```python
from build123d import *

# Parameters (mm, degrees)
SKETCH1_W               = 76.2
SKETCH1_H               = 25.4
SKETCH1_W_2             = 69.85
SKETCH1_H_2             = 19.05
EXTRUDE_THIN1_DEPTH     = 73.025
SKETCH2_W               = 63.5
SKETCH2_H               = 12.7
CUT_EXTRUDE1_DEPTH      = 26.4
SKETCH3_R               = 2.4892
CUT_EXTRUDE2_DEPTH      = 1
CUT_EXTRUDE2_DEPTH_BACK = 77.2
SKETCH4_R               = 6.35
CUT_EXTRUDE3_DEPTH      = 26.4


with BuildPart() as part:
    # Sketch1 → Extrude-Thin1 (new body, symmetric)
    with BuildSketch(Plane.XY):
        Rectangle(SKETCH1_W, SKETCH1_H)
        Rectangle(SKETCH1_W_2, SKETCH1_H_2, mode=Mode.SUBTRACT)
    extrude(amount=EXTRUDE_THIN1_DEPTH, both=True)

    # Sketch2 → Cut-Extrude1 (cut, through all)
    with BuildSketch(Plane.XZ.offset(12.7)):
        with Locations((0, -66.675)):
            Rectangle(SKETCH2_W, SKETCH2_H)
        with Locations((0, 66.675)):
            Rectangle(SKETCH2_W, SKETCH2_H)
    extrude(amount=-CUT_EXTRUDE1_DEPTH, mode=Mode.SUBTRACT)

    # Sketch3 → Cut-Extrude2 (cut, two sides)
    with BuildSketch(Plane(origin=(38.1, 0, 0), x_dir=(0, 0, -1), z_dir=(1, 0, 0))) as cut_extrude2_sk:
        with Locations((60.325, 7.62)):
            Circle(SKETCH3_R)
        with Locations((34.925, 7.62)):
            Circle(SKETCH3_R)
        with Locations((-34.925, 7.62)):
            Circle(SKETCH3_R)
        with Locations((-60.325, 7.62)):
            Circle(SKETCH3_R)
    extrude(amount=CUT_EXTRUDE2_DEPTH, mode=Mode.SUBTRACT)
    extrude(cut_extrude2_sk.sketch, amount=-CUT_EXTRUDE2_DEPTH_BACK, mode=Mode.SUBTRACT)

    # Sketch4 → Cut-Extrude3 (cut, through all)
    with BuildSketch(Plane.XZ.offset(12.7)):
        with Locations((0, 9.525)):
            Circle(SKETCH4_R)
    extrude(amount=-CUT_EXTRUDE3_DEPTH, mode=Mode.SUBTRACT)


solid = part.part
```
The listing builds one solid part. Answer for the finished solid, in the listing's coordinates (mm). A direction names the side the tool comes from. Round coordinates to 2 decimals unless told otherwise and drop trailing zeros. Write each loop counter-clockwise with the first axis right and the second up, starting at its lowest first coordinate (ties: lowest second). Pieces come first, ordered by that corner, then holes. Notation, with made-up numbers: (3.25, -19) -> (29.25, -19) arc R23 ccw to (29.25, 11) -> close; hole circle Ø10 at (52, -38). An arc over 180 degrees is marked (long way). Use CSV: the item, a comma, the result in double quotes. Start each with the question number.
(1) Section A-A on x = 0 is taken. Give the vertices of the cut face in (y, z) (3 decimals).
(2) Section B-B on z = -49 is taken. Give the vertices of the cut face in (x, y) (3 decimals).
(3) Each of these flat-tipped pins is pushed along its axis until it touches: pin 1 (1.6 mm diameter, centred on x = 1.5, y = -11.5, fed in from +Z) (3 decimals); pin 2 (0.8 mm diameter, centred on x = -9, y = 11.5, fed in from -Z) (3 decimals). Where does it stop, or does it pass through?
(4) Which of the six approach directions +Z, -Z, +X, -X, +Y, -Y give full straight-line access (tool end or side, diameter ignored) to faces 4 (the face through (34.925, 0, 1)), 5 (the face through (-31.75, 11, -67)), 6 (the face through (-36, 0, 73.025)), 7 (the face through (-31.75, 11, 67))?
(5) Consider L1, parallel to X at y = -3.5, z = 62.5 (3 decimals); L2, parallel to Y at x = -15.5, z = -17.5 (3 decimals); L3, parallel to X at y = 9.75, z = 65.5. Determine where each line is inside the solid, lowest interval first. Write a range as from..to.
(6) Section C-C on y = -5.5 is taken. Give the vertices of the cut face in (x, z) (3 decimals), then the cut area to 3 significant figures.
(7) Section D-D on x = -29 is taken. Give the vertices of the cut face in (y, z) (3 decimals), then the cut area to 3 significant figures.
(8) The mould has two halves that part along X. Classify faces 1 (the face through (3, 10, 59.6)), 2 (the face through (38.1, 0, 1)), 3 (the face through (-1.377, -11.135, 3.326)): released by +X, released by -X, zero draft, split by the parting line, or undercut.
A:
1,outline,"(-12.7, -60.325) -> (-9.525, -60.325) -> (-9.525, 3.175) -> (-12.7, 3.175) -> close; (-12.7, 15.875) -> (-9.525, 15.875) -> (-9.525, 60.325) -> (-12.7, 60.325) -> close; (9.525, -58.723) arc R2.489 cw to (10.109, -60.325) -> (12.7, -60.325) -> (12.7, 3.175) -> (9.525, 3.175) -> (9.525, -33.323) arc R2.489 cw to (9.525, -36.527) -> close; (9.525, 15.875) -> (12.7, 15.875) -> (12.7, 60.325) -> (10.109, 60.325) arc R2.489 cw to (9.525, 58.723) -> (9.525, 36.527) arc R2.489 cw to (9.525, 33.323) -> close"
2,outline,"(-38.1, -12.7) -> (38.1, -12.7) -> (38.1, 12.7) -> (-38.1, 12.7) -> close; hole (-34.925, -9.525) -> (34.925, -9.525) -> (34.925, 9.525) -> (-34.925, 9.525) -> close"
3,pin 1,"stops at z = 60.325"
3,pin 2,"stops at z = -60.325"
4,face 4,"+Z, -Z"
4,face 5,"-Z, +Y, -Y"
4,face 6,"+Z, +X, -X, +Y, -Y"
4,face 7,"+Z, +Y, -Y"
5,L1,"x = -38.1..-34.925, 34.925..38.1"
5,L2,"y = -12.7..-9.525, 9.525..12.7"
5,L3,"x = -38.1..-31.75, 31.75..38.1"
6,outline,"(-38.1, -73.025) -> (-34.925, -73.025) -> (-34.925, 73.025) -> (-38.1, 73.025) -> close; (34.925, -73.025) -> (38.1, -73.025) -> (38.1, 73.025) -> (34.925, 73.025) -> close"
6,area,"927 mm²"
7,outline,"(-12.7, -60.325) -> (-9.525, -60.325) -> (-9.525, 60.325) -> (-12.7, 60.325) -> close; (9.525, -58.723) arc R2.489 cw to (10.109, -60.325) -> (12.7, -60.325) -> (12.7, 60.325) -> (10.109, 60.325) arc R2.489 cw to (9.525, 58.723) -> (9.525, 36.527) arc R2.489 cw to (9.525, 33.323) -> (9.525, -33.323) arc R2.489 cw to (9.525, -36.527) -> close"
7,area,"762 mm²"
8,face 1,"zero draft"
8,face 2,"released by +X"
8,face 3,"undercut"
